from build123d import *

# Parameters (mm, degrees)
SKETCH1_W           = 90
SKETCH1_H           = 64
BOSS_EXTRUDE1_DEPTH = 33
SKETCH2_W           = 26
SKETCH2_H           = 14
CUT_EXTRUDE1_DEPTH  = 102.05938848
BOSS_EXTRUDE2_DEPTH = 24
SKETCH4_W           = 86.893013234
SKETCH4_H           = 16
CUT_EXTRUDE2_DEPTH  = 25
SKETCH6_W           = 28
SKETCH6_H           = 16
CUT_EXTRUDE3_DEPTH  = 40


with BuildPart() as part:
    # Sketch1 → Boss-Extrude1 (new body)
    with BuildSketch(Plane(origin=(0, 0, 0), x_dir=(1, 0, 0), z_dir=(0, 1, 0))):
        Rectangle(SKETCH1_W, SKETCH1_H)
    extrude(amount=BOSS_EXTRUDE1_DEPTH)

    # Sketch2 → Cut-Extrude1 (cut, through all)
    with BuildSketch(Plane(origin=(45, 0, 0), x_dir=(0, 0, -1), z_dir=(1, 0, 0))):
        with Locations((0, 7)):
            Rectangle(SKETCH2_W, SKETCH2_H)
    extrude(amount=-CUT_EXTRUDE1_DEPTH, mode=Mode.SUBTRACT)

    # Sketch3 → Boss-Extrude2 (add, symmetric)
    with BuildSketch(Plane.XY):
        with BuildLine():
            Line((0, 50), (0, 33))
            Line((0, 33), (45, 33))
            Line((45, 33), (30, 70))
            Line((30, 70), (20, 70))
            ThreePointArc((20, 70), (14.142135624, 55.857864376), (0, 50))
        make_face()
    boss_extrude2 = extrude(amount=BOSS_EXTRUDE2_DEPTH, both=True)

    # Mirror2: Boss-Extrude2 across plane
    add(boss_extrude2.mirror(Plane(origin=(0, 0, 0), x_dir=(0, 0, 1), z_dir=(1, 0, 0))))

    # Sketch4 → Cut-Extrude2 (cut)
    with BuildSketch(Plane(origin=(0, 70, 0), x_dir=(1, 0, 0), z_dir=(0, 1, 0))):
        Rectangle(SKETCH4_W, SKETCH4_H)
    extrude(amount=-CUT_EXTRUDE2_DEPTH, mode=Mode.SUBTRACT)

    # Sketch6 → Cut-Extrude3 (cut)
    with BuildSketch(Plane(origin=(0, 70, 0), x_dir=(1, 0, 0), z_dir=(0, 1, 0))):
        with Locations((0.173717363, -24)):
            Rectangle(SKETCH6_W, SKETCH6_H)
    cut_extrude3 = extrude(amount=-CUT_EXTRUDE3_DEPTH, mode=Mode.SUBTRACT)

    # Mirror3: Cut-Extrude3 across plane
    add(cut_extrude3.mirror(Plane.XY), mode=Mode.SUBTRACT)


solid = part.part
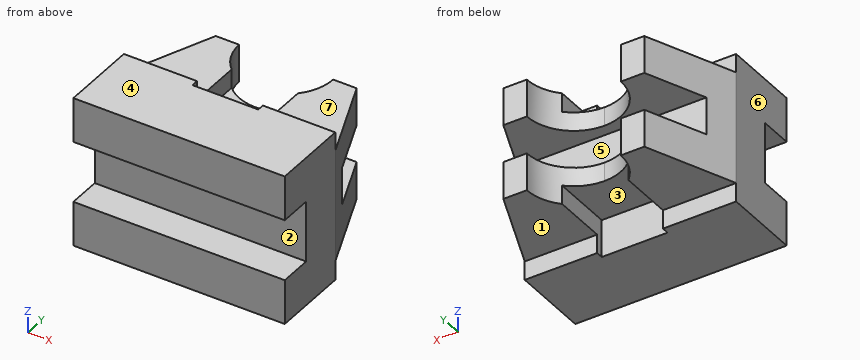
Check sheet for the modelled part. Datum: model origin and axes. Units: mm. Face numbers are marked on the shaded views. A direction names the side the tool comes from. Give positions to 0.01 mm unless a question says otherwise; leave off trailing zeros. Loops run counter-clockwise (first coordinate to the right, second up) from the corner with the lowest first, then second, coordinate; pieces in that order, holes last. Notation, with made-up numbers: M 4.5,63.5 L 41.5,63.5 A20 cw 41.5,84.5 Z; hole C -17,-1 d10. An arc over 180 degrees is marked long. Return JSON: item names as keys, results as strings. Group by question number.
1. Thickness scan on L1, parallel to Z at x = -5.5, y = 46; L2, parallel to Z at x = -27.5, y = 61; L3, parallel to Y at x = 30, z = 12.5. Record the ranges inside material, lowest first.
2. Cross-section at B-B on x = -23. Record the boundary of the cut face in (y, z), plus the area to 3 significant figures.
3. Cross-section at C-C on z = -10.5. Record the boundary of the cut face in (x, y).
4. Mould release check, pull along Z, two halves, no side actions. Record for the marked faces 5, 6 and 7: released by +Z, released by -Z, zero draft, split by the parting line, or undercut.
5. Tool access check on the marked faces 1, 2, 3 and 4. Record the directions out of +Z, -Z, +X, -X, +Y, -Y that give a thin tool (end or side, any length) a straight path to the whole face; none if there is none.
6. Cross-section at D-D on y = 59. Record the boundary of the cut face in (x, z).
7. Cross-section at A-A on y = 8. Record the boundary of the cut face in (x, z), plus the area to 3 significant figures.
8. Go/stop test with flat-tipped pins: pin 1 (4 mm diameter, centred on x = -31.5, z = 27.5, fed in from +Y); pin 2 (1.5 mm diameter, centred on x = -2.5, z = 8.5, fed in from -Y); pin 3 (2 mm diameter, centred on x = -1, z = -14.5, fed in from -Y); pin 4 (13 mm diameter, centred on x = 6.5, z = -22, fed in from +Y). Record where each tip stops, or that it passes through.
Return value:
{
 "1": {"L1": "-16 to -8, 8 to 16", "L2": "-24 to -8, 8 to 24", "L3": "14 to 70"},
 "2": {"outline": "M 0,-32 L 33,-32 L 33,-24 L 70,-24 L 70,-8 L 45,-8 L 45,8 L 70,8 L 70,24 L 33,24 L 33,32 L 0,32 L 0,13 L 14,13 L 14,-13 L 0,-13 Z", "area": "3,120 mm^2"},
 "3": {"outline": "M -45,14 L 45,14 L 45,33 L 30,70 L 20,70 A20 cw -20,70 L -30,70 L -45,33 Z"},
 "4": {"face 5": "undercut", "face 6": "zero draft", "face 7": "released by +Z"},
 "5": {"face 1": "-Z, +X, -X, +Y", "face 2": "+X, -X, -Y", "face 3": "-Z, +Y", "face 4": "+Z, +X, -X, +Y, -Y"},
 "6": {"outline": "M -34.46,-24 L -16.7,-24 L -16.7,-8 L -34.46,-8 Z; M -34.46,8 L -16.7,8 L -16.7,24 L -34.46,24 Z; M 16.7,-24 L 34.46,-24 L 34.46,-8 L 16.7,-8 Z; M 16.7,8 L 34.46,8 L 34.46,24 L 16.7,24 Z"},
 "7": {"outline": "M -45,-32 L 45,-32 L 45,-13 L -45,-13 Z; M -45,13 L 45,13 L 45,32 L -45,32 Z", "area": "3,420 mm^2"},
 "8": {"pin 1": "y = 33", "pin 2": "y = 14", "pin 3": "y = 0", "pin 4": "y = 52.14"}
}
